```python
from build123d import *

# Parameters (mm, degrees)
F0_W      = 50
F0_H      = 50
F1_DEPTH  = 30
F4_R      = 1.75
F5_DEPTH  = 50.001
F6_R      = 1.75
F7_DEPTH  = 50.001
F8_R      = 1.75
F9_DEPTH  = 20.105212
F11_R     = 5
F12_DEPTH = 20
F13_R     = 3


with BuildPart() as f1:
    # F0 (on Top) → F1 (new body)
    with BuildSketch(Plane.XY):
        Rectangle(F0_W, F0_H)
    extrude(amount=F1_DEPTH)

    # F2 (on Front) → F3 (revolve, cut)
    with BuildSketch(Plane.XZ):
        with BuildLine():
            Line((0, 265), (0, 15))
            ThreePointArc((0, 15), (125, 140), (0, 265))
        make_face()
    revolve(axis=Axis((0, 0, 140), (0, 0, 1)), mode=Mode.SUBTRACT)

    # F4 (on face) → F5 (cut, through all)
    with BuildSketch(Plane(origin=(-25, 0, 0), x_dir=(0, -1, 0), z_dir=(-1, 0, 0))):
        with Locations((-6.25, 12.17)):
            Circle(F4_R)
        with Locations((6.25, 12.17)):
            Circle(F4_R)
    extrude(amount=-F5_DEPTH, mode=Mode.SUBTRACT)

    # F6 (on face) → F7 (cut, through all)
    with BuildSketch(Plane.XZ.offset(25)):
        with Locations((-6.25, 12.17)):
            Circle(F6_R)
        with Locations((6.25, 12.17)):
            Circle(F6_R)
    extrude(amount=-F7_DEPTH, mode=Mode.SUBTRACT)

    # F8 (on Top) → F9 (cut, through all)
    with BuildSketch(Plane.XY):
        with Locations((17.5, 17.5)):
            Circle(F8_R)
        with Locations((17.5, -17.5)):
            Circle(F8_R)
        with Locations((-17.5, 17.5)):
            Circle(F8_R)
        with Locations((-17.5, -17.5)):
            Circle(F8_R)
    extrude(amount=F9_DEPTH, mode=Mode.SUBTRACT)

    # F11 (on offset) → F12 (cut)
    with BuildSketch(Plane.XY.offset(30)):
        with Locations((-17.5, 17.5)):
            Circle(F11_R)
        with Locations((-17.5, -17.5)):
            Circle(F11_R)
        with Locations((17.5, 17.5)):
            Circle(F11_R)
        with Locations((17.5, -17.5)):
            Circle(F11_R)
    extrude(amount=-F12_DEPTH, mode=Mode.SUBTRACT)

    # F13
    f13_edges = [f1.edges().sort_by_distance(p)[0] for p in [
        (-25, 0, 0),
        (0, -25, 0),
        (25, 0, 0),
        (0, 25, 0),
        (25, -25, 10.052106),
        (25, 25, 10.052106),
        (-25, 25, 10.052106),
        (-25, -25, 10.052106),
    ]]
    fillet(f13_edges, radius=F13_R)


solid = f1.part
```
The listing builds one solid part. Answer for the finished solid, in the listing's coordinates (mm). A direction names the side the tool comes from. Give positions to 0.01 mm unless a question says otherwise; leave off trailing zeros. Order: outer loops, then holes, each group sorted by start corner. A loop starts at its lowest first (then second) coordinate and runs counter-clockwise, first axis right, second up. Notation, with made-up numbers: (-20.5, -13.75) -> (30.5, -13.75) arc R25 ccw to (30.5, 3.25) -> close; hole circle Ø11 at (78, 3.25). An arc over 180 degrees is marked (long way). Write each question's results on one line, items separated by ' | '.
Q1. Determine the mould class of faces 3 (the face through (24.1, 0.31, 0.86)), 4 (the face through (-24.14, 24.1, 11.49)), 5 (the face through (-0.1, -4.5, 12.2)), 6 (the face through (-4.581, -15.756, 12.696)) for opening direction X: pulls with the +X half, pulls with the -X half, needs draft (parallel to the pull), parting line crosses it, or undercut.
Checked values:
face 3: pulls with the +X half | face 4: pulls with the -X half | face 5: needs draft | face 6: undercut
Q2. Straight lines are drawn through the part: probe 1 along Y at (x, z) = (-17.75, 12.17); probe 2 along Y at (x, z) = (-0.5, 12.17); probe 3 along X at (y, z) = (-17.5, 8.25). For each, find the intervals that lie inside material, in ascending order. Write a range as from..to.
Checked values:
probe 1: y = -25..-22.49, -12.51..-8, -4.5..4.5, 8..12.51, 22.49..25 | probe 2: y = -25..-8, -4.5..4.5, 8..25 | probe 3: x = -25..-19.25, -15.75..15.75, 19.25..25
Q3. The part is cut by section A-A, the plane z = 8. Give the vertices of the cut face in (x, y).
Checked values:
outline: (-25, -22) arc R3 ccw to (-22, -25) -> (22, -25) arc R3 ccw to (25, -22) -> (25, 22) arc R3 ccw to (22, 25) -> (-22, 25) arc R3 ccw to (-25, 22) -> close; hole circle Ø3.5 at (-17.5, -17.5); hole circle Ø3.5 at (-17.5, 17.5); hole circle Ø3.5 at (17.5, -17.5); hole circle Ø3.5 at (17.5, 17.5)
Q4. Which of the six approach directions +Z, -Z, +X, -X, +Y, -Y give full straight-line access (tool end or side, diameter ignored) to faces 1 (the face through (-18.79, 18.68, 4.93)), 2 (the face through (17, 15, 10))?
Checked values:
face 1: +Z, -Z | face 2: +Z
Q5. Each of these flat-tipped pins is pushed along its axis until it touches: P1, Ø2, axis at y = -6.25, z = 12.17, coming from the -X side; P2, Ø11, axis at x = 17.5, y = -17.5, coming from the +Z side; P3, Ø2, axis at x = 11.5, y = -16, coming from the +Z side; P4, Ø2, axis at x = 19.5, y = 9, coming from the +Z side. Where does it stop, or does it pass through?
Checked values:
P1: passes through | P2: stops at z = 18.72 | P3: stops at z = 16.73 | P4: stops at z = 17.04
Q6. The part is cut by section D-D, the plane z = 16.25. Give the vertices of the cut face in (x, y).
Checked values:
outline: (-25, -22) arc R3 ccw to (-22, -25) -> (22, -25) arc R3 ccw to (25, -22) -> (25, 22) arc R3 ccw to (22, 25) -> (-22, 25) arc R3 ccw to (-25, 22) -> close; hole circle Ø10 at (-17.5, -17.5); hole circle Ø10 at (-17.5, 17.5); hole circle Ø35.27 at (0, 0); hole circle Ø10 at (17.5, -17.5); hole circle Ø10 at (17.5, 17.5)
Q7. The part is cut by section B-B, the plane x = -17.5. Give the vertices of the cut face in (y, z).
Checked values:
outline: (-25, 3) arc R3 ccw to (-22, 0) -> (-19.25, 0) -> (-19.25, 10) -> (-22.5, 10) -> (-22.5, 18.29) arc R123.77 cw to (-25, 18.78) -> close; (-15.75, 0) -> (15.75, 0) -> (15.75, 10) -> (12.5, 10) -> (12.5, 16.86) arc R123.77 cw to (-12.5, 16.86) -> (-12.5, 10) -> (-15.75, 10) -> close; (19.25, 0) -> (22, 0) arc R3 ccw to (25, 3) -> (25, 18.78) arc R123.77 cw to (22.5, 18.29) -> (22.5, 10) -> (19.25, 10) -> close; hole circle Ø3.5 at (-6.25, 12.17); hole circle Ø3.5 at (6.25, 12.17)
